from build123d import *

# Parameters (mm, degrees)
EXTRUDE_1_DEPTH     = 9
EXTRUDE_2_DEPTH     = 225
EXTRUDE_3_DEPTH     = 9
SKETCH_6_R          = 9.5
CUT_EXTRUDE_3_DEPTH = 3.25
CUT_EXTRUDE_START   = -3.25
SKETCH_7_R          = 9.5
CUT_EXTRUDE_4_DEPTH = 3.25
EXTRUDE_4_DEPTH     = 175
CUT_EXTRUDE_5_REACH = 246.729
SKETCH_10_R         = 8
SKETCH_11_R         = 5
CUT_EXTRUDE_6_DEPTH = 10


with BuildPart() as part:
    # 草图1 → 凸台-拉伸1 (new body)
    with BuildSketch(Plane.XY):
        with BuildLine():
            Line((-25.5, 40), (25.5, 40))
            ThreePointArc((25.5, 40), (27.621320344, 39.121320344), (28.5, 37))
            Line((28.5, 37), (28.5, -40))
            Line((28.5, -40), (-28.5, -40))
            Line((-28.5, -40), (-28.5, 37))
            ThreePointArc((-28.5, 37), (-27.621320344, 39.121320344), (-25.5, 40))
        make_face()
    extrude(amount=EXTRUDE_1_DEPTH)

    # 草图2 → 凸台-拉伸2 (add)
    with BuildSketch(Plane.XY.offset(9)):
        Polygon((-20, -40), (-12.1, -40), (-12.1, -33.8), (-7.9, -33.8), (-7.9, -40), (7.9, -40), (7.9, -33.8), (12.1, -33.8), (12.1, -40), (20, -40), (20, -32.1), (13.8, -32.1), (13.8, -27.9), (20, -27.9), (20, -20), (12.1, -20), (12.1, -26.2), (7.9, -26.2), (7.9, -20), (-7.9, -20), (-7.9, -26.2), (-12.1, -26.2), (-12.1, -20), (-20, -20), (-20, -27.9), (-13.8, -27.9), (-13.8, -32.1), (-20, -32.1), align=None)
    extrude(amount=EXTRUDE_2_DEPTH)

    # 草图3 → 凸台-拉伸3 (add)
    with BuildSketch(Plane.XY.offset(234)):
        with BuildLine():
            Line((-21, -40), (21, -40))
            Line((21, -40), (21, 22))
            ThreePointArc((21, 22), (20.121320344, 24.121320344), (18, 25))
            Line((18, 25), (-18, 25))
            ThreePointArc((-18, 25), (-20.121320344, 24.121320344), (-21, 22))
            Line((-21, 22), (-21, -40))
        make_face()
    extrude(amount=EXTRUDE_3_DEPTH)

    # 草图6 → 切除-拉伸3 (cut)
    with BuildSketch(Plane.XY.offset(243)):
        with Locations((0, 10)):
            Circle(SKETCH_6_R)
    extrude(amount=-CUT_EXTRUDE_3_DEPTH, mode=Mode.SUBTRACT)

    # 草图7 → 切除-拉伸4 (cut)
    with BuildSketch(Plane(origin=(0, 0, 234), x_dir=(-1, 0, 0), z_dir=(0, 0, -1)).offset(CUT_EXTRUDE_START)):
        with Locations(Location((0, 10, 0), (0, 0, 180))):
            Circle(SKETCH_7_R)
    extrude(amount=CUT_EXTRUDE_4_DEPTH, mode=Mode.SUBTRACT)

    # 草图8 → 凸台-拉伸4 (add)
    with BuildSketch(Plane(origin=(0, 0, 234), x_dir=(-1, 0, 0), z_dir=(0, 0, -1))):
        Polygon((-6, -20), (6, -20), (6, -14.65), (4.5, -14.65), (4.5, -13.65), (6, -13.65), (6, -12.15), (-6, -12.15), (-6, -13.65), (-4.5, -13.65), (-4.5, -14.65), (-6, -14.65), align=None)
    extrude(amount=EXTRUDE_4_DEPTH)

    # 草图10 → 切除-拉伸5 (cut, up to next)
    with BuildSketch(Plane.XY.offset(239.75), mode=Mode.PRIVATE) as cut_extrude_5_sk1:
        with Locations((0, 10)):
            Circle(SKETCH_10_R)
    cut_extrude_5_tool1 = extrude(cut_extrude_5_sk1.sketch, amount=-CUT_EXTRUDE_5_REACH, mode=Mode.PRIVATE) & part.part
    add(cut_extrude_5_tool1.solids().sort_by_distance((0, 10, 239.75))[0], mode=Mode.SUBTRACT)

    # 草图11 → 切除-拉伸6 (cut)
    with BuildSketch(Plane(origin=(0, 0, 0), x_dir=(-1, 0, 0), z_dir=(0, 0, -1))):
        with Locations((0, 10)):
            Circle(SKETCH_11_R)
    extrude(amount=-CUT_EXTRUDE_6_DEPTH, mode=Mode.SUBTRACT)


solid = part.part
Build history of the part. All positions in model axes, mm. A direction names the side the tool comes from. Give positions to 0.01 mm unless a question says otherwise; leave off trailing zeros. Order: outer loops, then holes, each group sorted by start corner. A loop starts at its lowest first (then second) coordinate and runs counter-clockwise, first axis right, second up. Notation, with made-up numbers: M 45.5,55 L 98.5,55 A13 ccw 98.5,65 Z; hole C 72.5,15 d3. An arc over 180 degrees is marked long. Use one line per item in the form item = value.
1) Drop flat-ended pins along their axis: pin 1 (1.3 mm diameter, centred on x = -9.5, y = -36, fed in from -Z); pin 2 (8 mm diameter, centred on y = -21.5, z = 71, fed in from +X); pin 3 (3 mm diameter, centred on x = 17, z = 168, fed in from +Y); pin 4 (4.5 mm diameter, centred on y = -30, z = 160.5, fed in from -X). Give the stop position or say it passes through.
Calculated:
pin_1 = 0
pin_2 = 20
pin_3 = -20
pin_4 = -20
2) Tool access for faces 1 (the face through (10, -26.2, 120)), 2 (the face through (-1.73, 2.19, 238.52)), 3 (the face through (-21, -9, 238)), 4 (the face through (21, -9, 238)): list every direction of +Z, -Z, +X, -X, +Y, -Y with a clear straight run to the whole face (end or side of a thin tool).
Calculated:
face_1 = +Y
face_2 = +Z
face_3 = +Z, -X, +Y, -Y
face_4 = +Z, +X, +Y, -Y
3) Two-plate mould, pull along Z, no slides. Class faces 5 (the face through (-4.3, 3, 239.75)), 6 (the face through (28.5, -1, 4)), 7 (the face through (12.1, -23, 120)), 8 (the face through (-16, -20, 120)): released by +Z, released by -Z, zero draft, split by the parting line, or undercut.
Calculated:
face_5 = released by +Z
face_6 = zero draft
face_7 = undercut
face_8 = undercut
4) Probe probe 1 along X at (y, z) = (-24, 100); probe 2 along Y at (x, z) = (-16, 56.5); probe 3 along Z at (x, y) = (7, 6). List the from-to ranges inside material, lowest first.
Calculated:
probe_1 = -20 to -12.1, -7.9 to 7.9, 12.1 to 20
probe_2 = -40 to -32.1, -27.9 to -20
probe_3 = 0 to 9, 237.25 to 239.75
5) Saw through at A-A (y = 10). Give the cut face in (x, z), plus the area to 4 significant figures.
Calculated:
outline = M -28.5,0 L -5,0 L -5,9 L -28.5,9 Z; M -21,234 L -9.5,234 L -9.5,237.25 L -8,237.25 L -8,239.75 L -9.5,239.75 L -9.5,243 L -21,243 Z; M 5,0 L 28.5,0 L 28.5,9 L 5,9 Z; M 8,237.25 L 9.5,237.25 L 9.5,234 L 21,234 L 21,243 L 9.5,243 L 9.5,239.75 L 8,239.75 Z
area = 637.5 mm2
6) Saw through at C-C (z = 24.5). Give the cut face in (x, y), plus the area to 3 significant figures.
Calculated:
outline = M -20,-40 L -12.1,-40 L -12.1,-33.8 L -7.9,-33.8 L -7.9,-40 L 7.9,-40 L 7.9,-33.8 L 12.1,-33.8 L 12.1,-40 L 20,-40 L 20,-32.1 L 13.8,-32.1 L 13.8,-27.9 L 20,-27.9 L 20,-20 L 12.1,-20 L 12.1,-26.2 L 7.9,-26.2 L 7.9,-20 L -7.9,-20 L -7.9,-26.2 L -12.1,-26.2 L -12.1,-20 L -20,-20 L -20,-27.9 L -13.8,-27.9 L -13.8,-32.1 L -20,-32.1 Z
area = 644 mm2
7) Saw through at B-B (x = 0). Give the cut face in (y, z), plus the area to 3 significant figures.
Calculated:
outline = M -40,0 L 5,0 L 5,9 L -20,9 L -20,59 L -12.15,59 L -12.15,234 L 0.5,234 L 0.5,237.25 L 2,237.25 L 2,239.75 L 0.5,239.75 L 0.5,243 L -40,243 Z; M 15,0 L 40,0 L 40,9 L 15,9 Z; M 18,237.25 L 19.5,237.25 L 19.5,234 L 25,234 L 25,243 L 19.5,243 L 19.5,239.75 L 18,239.75 Z
area = 6,930 mm2
